Part model, mm, in its own coordinate system. Round coordinates to 2 decimals unless told otherwise and drop trailing zeros. Order: outer loops, then holes, each group sorted by start corner. A loop starts at its lowest first (then second) coordinate and runs counter-clockwise, first axis right, second up. Notation, with made-up numbers: (0.25, 82.5) -> (53.25, 82.5) arc R12 ccw to (53.25, 92.5) -> close; hole circle Ø9 at (37, 2). An arc over 180 degrees is marked (long way). Use CSV: the item, a comma, the result in double quotes.
```python
from build123d import *

# Parameters (mm, degrees)
SKETCH1_W                    = 60.96
SKETCH1_H                    = 10
BASE_FLANGE1_DEPTH           = 1.1684
EDGE_FLANGE1_STRIP_W         = 7.0104
EDGE_FLANGE1_STRIP_H         = 1.1684
EDGE_FLANGE1_STRIP_CUT_DEPTH = 60.96
EDGE_FLANGE1_DEPTH           = 60.96
TAP_DRILL_FOR_M3X0_5_TAP1_D  = 2.5
FILLET1_DEPTH                = 60.96
FILLET1_2_DEPTH              = 60.96
FILLET1_START                = -2
FILLET1_3_DEPTH              = 3


with BuildPart() as part:
    # Base-Flange1: sheet metal written as solids
    # Sketch1 → Base-Flange1 (new body)
    with BuildSketch(Plane(origin=(0, 0, 0), x_dir=(1, 0, 0), z_dir=(0, 1, 0))):
        with Locations((30.48, 5)):
            Rectangle(SKETCH1_W, SKETCH1_H)
    extrude(amount=-BASE_FLANGE1_DEPTH)

    # Edge-Flange1: sheet metal written as solids
    # Edge-Flange1 strip (on a plane across the edge) → Edge-Flange1 strip cut (cut)
    with BuildSketch(Plane(origin=(0, -1.1684, -10), x_dir=(0, 0, 1), z_dir=(1, 0, 0))):
        with Locations((-1.1684, -0.5842)):
            Rectangle(EDGE_FLANGE1_STRIP_W, EDGE_FLANGE1_STRIP_H)
    extrude(amount=EDGE_FLANGE1_STRIP_CUT_DEPTH, mode=Mode.SUBTRACT)

    # Edge-Flange1 section (on a plane across the edge) → Edge-Flange1 (add)
    with BuildSketch(Plane(origin=(0, -1.1684, -10), x_dir=(0, 0, 1), z_dir=(1, 0, 0))):
        with BuildLine():
            Line((0, 1.1684), (0, 9))
            Line((0, 9), (1.1684, 9))
            Line((1.1684, 9), (1.1684, 1.1684))
            ThreePointArc((1.1684, 1.1684), (1.510616437, 0.342216437), (2.3368, 0))
            Line((2.3368, 0), (2.3368, -1.1684))
            ThreePointArc((2.3368, -1.1684), (0.684432874, -0.483967126), (0, 1.1684))
        make_face()
    extrude(amount=EDGE_FLANGE1_DEPTH)

    # Tap Drill for M3x0.5 Tap1 (through all)
    with Locations(Plane(origin=(0, -1.1684, 0), x_dir=(-1, 0, 0), z_dir=(0, -1, 0))):
        with Locations((-2.55, 5.94), (-22.87, 5.94), (-43.19, 5.94)):
            Hole(TAP_DRILL_FOR_M3X0_5_TAP1_D / 2)

    # Fillet1: read off the stored shape, not the designer's step
    # Fillet1 outline → Fillet1 (cut)
    with BuildSketch(Plane.YZ):
        with BuildLine():
            ThreePointArc((-2.3368, -10), (-1.731991655, -9.920375471), (-1.1684, -9.686928163))
            Line((-1.1684, -9.686928163), (-1.1684, -7.6632))
            ThreePointArc((-1.1684, -7.6632), (-1.510616437, -8.489383563), (-2.3368, -8.8316))
            Line((-2.3368, -8.8316), (-10.1684, -8.8316))
            Line((-10.1684, -8.8316), (-10.1684, -10))
            Line((-10.1684, -10), (-2.3368, -10))
        make_face()
    extrude(amount=FILLET1_DEPTH, mode=Mode.SUBTRACT)

    # Fillet1 2 outline → Fillet1 2 (add)
    with BuildSketch(Plane.YZ):
        with BuildLine():
            Line((0, -18.247777642), (0, -7.6632))
            ThreePointArc((0, -7.6632), (-0.313071837, -8.8316), (-1.1684, -9.686928163))
            Line((-1.1684, -9.686928163), (-1.1684, -18.247777642))
            Line((-1.1684, -18.247777642), (0, -18.247777642))
        make_face()
    extrude(amount=FILLET1_2_DEPTH)

    # Fillet1 3 outline → Fillet1 3 (cut)
    with BuildSketch(Plane(origin=(0, 0, 0), x_dir=(1, 0, 0), z_dir=(0, 1, 0)).offset(FILLET1_START)):
        with BuildLine():
            Line((60.96, 18.247777642), (56.96, 18.247777642))
            ThreePointArc((56.96, 18.247777642), (59.788427125, 17.076204767), (60.96, 14.247777642))
            Line((60.96, 14.247777642), (60.96, 18.247777642))
        make_face()
        with BuildLine():
            ThreePointArc((0, 14.247777642), (1.171572875, 17.076204767), (4, 18.247777642))
            Line((4, 18.247777642), (0, 18.247777642))
            Line((0, 18.247777642), (0, 14.247777642))
        make_face()
        with BuildLine():
            Line((60.96, 0), (60.96, 4))
            ThreePointArc((60.96, 4), (59.788427125, 1.171572875), (56.96, 0))
            Line((56.96, 0), (60.96, 0))
        make_face()
        with BuildLine():
            ThreePointArc((4, 0), (1.171572875, 1.171572875), (0, 4))
            Line((0, 4), (0, 0))
            Line((0, 0), (4, 0))
        make_face()
    extrude(amount=FILLET1_3_DEPTH, mode=Mode.SUBTRACT)


solid = part.part
```
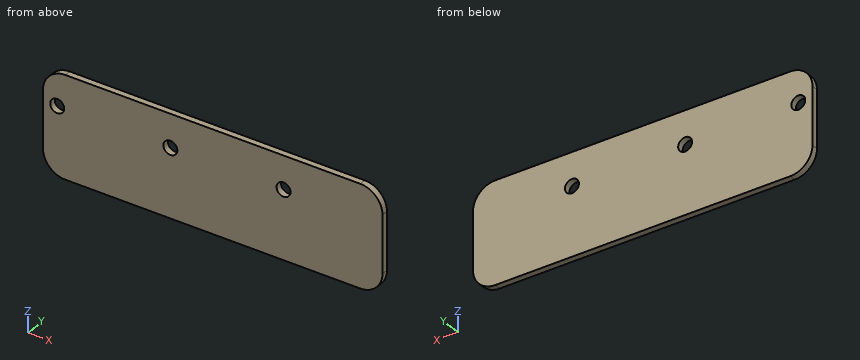
(1) Cut at A-A, the plane z = -5.94. Give the cut face in (x, y).
Reply:
outline,"(0, -1.17) -> (1.3, -1.17) -> (1.3, 0) -> (0, 0) -> close; (3.8, -1.17) -> (21.62, -1.17) -> (21.62, 0) -> (3.8, 0) -> close; (24.12, -1.17) -> (41.94, -1.17) -> (41.94, 0) -> (24.12, 0) -> close; (44.44, -1.17) -> (60.96, -1.17) -> (60.96, 0) -> (44.44, 0) -> close"
(2) Cut at B-B, the plane x = 43.19. Give the cut face in (y, z), then the cut area to 3 significant figures.
Reply:
outline,"(-1.17, -18.25) -> (0, -18.25) -> (0, -7.19) -> (-1.17, -7.19) -> close; (-1.17, -4.69) -> (0, -4.69) -> (0, 0) -> (-1.17, 0) -> close"
area,"18.4 mm2"
(3) Cut at D-D, the plane x = 2.55. Give the cut face in (y, z).
Reply:
outline,"(-1.17, -17.98) -> (0, -17.98) -> (0, -7.19) -> (-1.17, -7.19) -> close; (-1.17, -4.69) -> (0, -4.69) -> (0, -0.27) -> (-1.17, -0.27) -> close"
(4) Probe probe 1 along X at (y, z) = (-0.45, -5.94); probe 2 along Z at (x, y) = (22.87, -0.8); probe 3 along Z at (x, y) = (3.5, -0.5). List the from-to ranges inside material, lowest first. Write a range as [from, to].
Reply:
probe 1,"[0, 1.3], [3.8, 21.62], [24.12, 41.94], [44.44, 60.96]"
probe 2,"[-18.25, -7.19], [-4.69, 0]"
probe 3,"[-18.22, -6.75], [-5.13, -0.03]"
(5) Cut at C-C, the plane y = -0.9. Give the cut face in (x, z), then the cut area to 3 significant figures.
Reply:
outline,"(0, -14.25) arc R4 ccw to (4, -18.25) -> (56.96, -18.25) arc R4 ccw to (60.96, -14.25) -> (60.96, -4) arc R4 ccw to (56.96, 0) -> (4, 0) arc R4 ccw to (0, -4) -> close; hole circle Ø2.5 at (2.55, -5.94); hole circle Ø2.5 at (22.87, -5.94); hole circle Ø2.5 at (43.19, -5.94)"
area,"1,080 mm2"
(6) Drop a flat-ended pin along its axis: P1, Ø6, axis at x = 50, z = -14.5, coming from the +Y side. Give the stop position or say it passes through.
Reply:
P1,"y = 0"
